from build123d import *

# Parameters (mm, degrees)
F0_W        = 147.8525847197
F0_H        = 85.1719379425
F0_W_2      = 59.7309665754
F0_H_2      = 5.5306423455
F0_W_3      = 58.9935472235
F0_H_3      = 4.7932267189
F0_W_4      = 57.5187108479
F0_H_4      = 5.1619354635
F0_W_5      = 55.6751615368
F0_W_6      = 57.8874191269
F0_H_5      = 3.6870967597
F0_W_7      = 56.7812863737
F0_H_6      = 4.7932248563
F0_W_8      = 52.7254838962
F0_H_7      = 5.5306442082
F0_H_8      = 6.6367760301
F1_DEPTH    = 10.16
F2_T1_DEPTH = 147.3889774092
F3_R        = 5.08
F4_R        = 4.5031383634
F5_DEPTH    = 25.4


# Not quite as in the source:
# - a fillet or chamfer that OpenCascade refuses, or shapes differently, is made with other operations: its cross-section is extruded or revolved along the edge and cut away or added


with BuildPart() as f1:
    # F0 (on Top) → F1 (new body)
    with BuildSketch(Plane.XY):
        Rectangle(F0_W, F0_H)
        with Locations((-38.0981913768, -32.7256983146)):
            Rectangle(F0_W_2, F0_H_2, mode=Mode.SUBTRACT)
        with Locations((-38.4669010527, -18.7147296965)):
            Rectangle(F0_W_3, F0_H_3, mode=Mode.SUBTRACT)
        with Locations((32.6940652449, -32.5413448736)):
            Rectangle(F0_W_4, F0_H_4, mode=Mode.SUBTRACT)
        with Locations((31.7722905893, -18.7147296965)):
            Rectangle(F0_W_5, F0_H_3, mode=Mode.SUBTRACT)
        with Locations((-39.019965101, 16.4970448241)):
            Rectangle(F0_W_6, F0_H_5, mode=Mode.SUBTRACT)
        with Locations((-39.5730314776, 32.535915263)):
            Rectangle(F0_W_7, F0_H_6, mode=Mode.SUBTRACT)
        with Locations((29.1913239053, 17.4188185483)):
            Rectangle(F0_W_8, F0_H_7, mode=Mode.SUBTRACT)
        with Locations((29.1913239053, 32.3515608907)):
            Rectangle(F0_W_8, F0_H_8, mode=Mode.SUBTRACT)
    extrude(amount=F1_DEPTH)

    # F2: fillet of radius 12.7 on 1 edges, made by hand

    # F2_s2 → F2_t1 (cut)
    with BuildSketch(Plane.XZ.offset(-73.6944887046)):
        with BuildLine():
            ThreePointArc((-73.9262923598, 0), (-69.5150697233, 7.2973776994), (-61.4828844665, 10.16))
            Line((-61.4828844665, 10.16), (-73.9262923598, 10.16))
            Line((-73.9262923598, 10.16), (-73.9262923598, 0))
        make_face()
    extrude(amount=F2_T1_DEPTH, mode=Mode.SUBTRACT)

    # F3
    f3_edges = [f1.edges().sort_by_distance(p)[0] for p in [
        (6.221704, -42.585969, 10.16),
        (6.221704, 42.585969, 10.16),
        (-69.51507, 42.585969, 7.297378),
        (-69.51507, -42.585969, 7.297378),
    ]]
    fillet(f3_edges, radius=F3_R)

    # F4 (on face) → F5 (join)
    with BuildSketch(Plane.YZ.offset(73.9262923598)):
        with Locations((0, 5.0259334967)):
            Circle(F4_R)
    extrude(amount=F5_DEPTH)


solid = f1.part
Check sheet for the modelled part. Datum: model origin and axes. Units: mm. Give positions to 0.01 mm unless a question says otherwise; leave off trailing zeros. Order: outer loops, then holes, each group sorted by start corner. A loop starts at its lowest first (then second) coordinate and runs counter-clockwise, first axis right, second up. Notation, with made-up numbers: (46, 30) - (58, 30) arc R20 cw to (58, 35) - close; hole circle Ø9 at (73.5, 43.5). An arc over 180 degrees is marked (long way). Answer as CSV lines item,"result".
1. Section check C-C (y = 0). Record the boundary of the cut face in (x, z), then the cut area to 3 significant figures.
Result sheet:
outline,"(-73.93, 0) - (73.93, 0) - (73.93, 0.52) - (99.33, 0.52) - (99.33, 9.53) - (73.93, 9.53) - (73.93, 10.16) - (-61.48, 10.16) arc R12.7 ccw to start"
area,"1,700 mm²"
2. Mould release check, pull along Y, two halves, no side actions. Record for faces 1 (the face through (5, 1, 10.16)), 2 (the face through (-11.182, 33, 5)), 3 (the face through (86.45, -0.59, 9.49)), 4 (the face through (2, 42.586, 3)): released by +Y, released by -Y, zero draft, split by the parting line, or undercut.
Result sheet:
face 1,"zero draft"
face 2,"undercut"
face 3,"split by the parting line"
face 4,"released by +Y"
3. Section check D-D (x = 28). Record the boundary of the cut face in (y, z), then the cut area to 3 significant figures.
Result sheet:
outline,"(-42.59, 0) - (-35.12, 0) - (-35.12, 10.16) - (-37.51, 10.16) arc R5.08 ccw to (-42.59, 5.08) - close; (-29.96, 0) - (-21.11, 0) - (-21.11, 10.16) - (-29.96, 10.16) - close; (-16.32, 0) - (14.65, 0) - (14.65, 10.16) - (-16.32, 10.16) - close; (20.18, 0) - (29.03, 0) - (29.03, 10.16) - (20.18, 10.16) - close; (35.67, 0) - (42.59, 0) - (42.59, 5.08) arc R5.08 ccw to (37.51, 10.16) - (35.67, 10.16) - close"
area,"630 mm²"
4. Section check A-A (y = -19.5). Record the boundary of the cut face in (x, z).
Result sheet:
outline,"(-73.93, 0) - (-67.96, 0) - (-67.96, 8.38) arc R12.7 ccw to start; (-8.97, 0) - (3.93, 0) - (3.93, 10.16) - (-8.97, 10.16) - close; (59.61, 0) - (73.93, 0) - (73.93, 10.16) - (59.61, 10.16) - close"
5. Go/stop test with flat-tipped pins: P1, Ø3, axis at x = 21.5, z = 7, coming from the +Y side; P2, Ø4, axis at y = -18, z = 4, coming from the +X side; P3, Ø5.5, axis at y = -19.5, z = 3.5, coming from the -X side. Record where each tip stops, or that it passes through.
Result sheet:
P1,"y = 42.57"
P2,"x = 73.93"
P3,"x = -73.75"
6. Scan lines: probe 1 along Y at (x, z) = (-31.5, 2.25); probe 2 along Y at (x, z) = (48, 0.5); probe 3 along Y at (x, z) = (57, 6.75). Record each from-to range of solid material in increasing order. Write a range as from..to.
Result sheet:
probe 1,"-42.59..-35.49, -29.96..-21.11, -16.32..14.65, 18.34..30.14, 34.93..42.59"
probe 2,"-42.59..-35.12, -29.96..-21.11, -16.32..14.65, 20.18..29.03, 35.67..42.59"
probe 3,"-42.3..-35.12, -29.96..-21.11, -16.32..42.3"
7. Section check B-B (x = -50.5). Record the boundary of the cut face in (y, z), then the cut area to 3 significant figures.
Result sheet:
outline,"(-42.59, 0) - (-35.49, 0) - (-35.49, 10.16) - (-37.51, 10.16) arc R5.08 ccw to (-42.59, 5.08) - close; (-29.96, 0) - (-21.11, 0) - (-21.11, 10.16) - (-29.96, 10.16) - close; (-16.32, 0) - (14.65, 0) - (14.65, 10.16) - (-16.32, 10.16) - close; (18.34, 0) - (30.14, 0) - (30.14, 10.16) - (18.34, 10.16) - close; (34.93, 0) - (42.59, 0) - (42.59, 5.08) arc R5.08 ccw to (37.51, 10.16) - (34.93, 10.16) - close"
area,"663 mm²"
